from build123d import *

# Parameters (mm, degrees)
BOSS_EXTRU_1_DEPTH      = 5
ESQUISSE3_R             = 5
ENL_V_MAT_EXTRU_1_DEPTH = 10


with BuildPart() as part:
    # Esquisse2 → Boss.-Extru.1 (new body)
    with BuildSketch(Plane.XY):
        with BuildLine():
            Line((-8, -7.5), (-8, 7.5))
            ThreePointArc((-8, 7.5), (0, 15.5), (8, 7.5))
            Line((8, 7.5), (8, -7.5))
            ThreePointArc((8, -7.5), (0, -15.5), (-8, -7.5))
        make_face()
    extrude(amount=BOSS_EXTRU_1_DEPTH)

    # Esquisse3 → Enlèv. mat.-Extru.1 (cut)
    with BuildSketch(Plane.XY.offset(5)):
        Circle(ESQUISSE3_R)
    extrude(amount=-ENL_V_MAT_EXTRU_1_DEPTH, mode=Mode.SUBTRACT)


solid = part.part
Geometry: final body of the model. Coordinates: model frame, mm. Give positions to 0.01 mm unless a question says otherwise; leave off trailing zeros. Order: outer loops, then holes, each group sorted by start corner. A loop starts at its lowest first (then second) coordinate and runs counter-clockwise, first axis right, second up. Notation, with made-up numbers: (15.5, -15.5) -> (20.5, -15.5) arc R13 ccw to (20.5, -9.5) -> close; hole circle Ø2 at (56.5, 87.5). An arc over 180 degrees is marked (long way). Answer as a JSON object with one key per item and string values.
Q1. First-contact query: pin 1 (4 mm diameter, centred on x = 4, y = 8, fed in from -Z); pin 2 (1.5 mm diameter, centred on x = -5, z = 1.5, fed in from -Y); pin 3 (1.5 mm diameter, centred on x = -2, z = 1.5, fed in from -Y); pin 4 (1.5 mm diameter, centred on x = -2, z = 3.5, fed in from +Y). Flat tips, straight axial feed; report the tip coordinate or a pass-through.
Entries:
{"pin 1": "stops at z = 0", "pin 2": "stops at y = -14.28", "pin 3": "stops at y = -15.4", "pin 4": "stops at y = 15.4"}
Q2. Section A-A (y = 0). Output: boundary loops of the cut face in (x, z).
Entries:
{"outline": "(-8, 0) -> (-5, 0) -> (-5, 5) -> (-8, 5) -> close; (5, 0) -> (8, 0) -> (8, 5) -> (5, 5) -> close"}
Q3. Section B-B (x = 0). Output: boundary loops of the cut face in (y, z), plus the area to 3 significant figures.
Entries:
{"outline": "(-15.5, 0) -> (-5, 0) -> (-5, 5) -> (-15.5, 5) -> close; (5, 0) -> (15.5, 0) -> (15.5, 5) -> (5, 5) -> close", "area": "105 mm^2"}
Q4. Material intervals for probe 1 along Y at (x, z) = (0, 3.85); probe 2 along Y at (x, z) = (4.5, 1); probe 3 along X at (y, z) = (-2.5, 2.85), sorted ascending.
Entries:
{"probe 1": "y = -15.5 to -5, 5 to 15.5", "probe 2": "y = -14.11 to -2.18, 2.18 to 14.11", "probe 3": "x = -8 to -4.33, 4.33 to 8"}
Q5. Draft query along X for faces 1 (the cylindrical face through (-0.176, 15.498, 2.465)), 2 (the cylindrical face through (-1.08, -4.88, 2.54)), 3 (the flat face through (4, 4, 5)). Return one class per face: released by +X, released by -X, zero draft, split by the parting line, or undercut.
Entries:
{"face 1": "split by the parting line", "face 2": "undercut", "face 3": "zero draft"}
Q6. Section D-D (x = 6). Output: boundary loops of the cut face in (y, z).
Entries:
{"outline": "(-12.79, 0) -> (12.79, 0) -> (12.79, 5) -> (-12.79, 5) -> close"}
Q7. Section C-C (z = 0.55). Output: boundary loops of the cut face in (x, y).
Entries:
{"outline": "(-8, -7.5) arc R8 ccw to (8, -7.5) -> (8, 7.5) arc R8 ccw to (-8, 7.5) -> close; hole circle Ø10 at (0, 0)"}
